Answer from the drawing. Dimensions are ordinates in mm from the lowest x, y and z of the part. A direction names the side the tool comes from. Coordinates: 2 decimals unless noted, no trailing zeros. Write each loop counter-clockwise with the first axis right and the second up, starting at its lowest first coordinate (ties: lowest second). Pieces come first, ordered by that corner, then holes. Notation, with made-up numbers: M 0.25,-16 L 47.25,-16 A19 ccw 47.25,-9 Z; hole C -9,-15 d8. An arc over 180 degrees is marked long. Put each result on its own line as item: value. Start each with the question number.
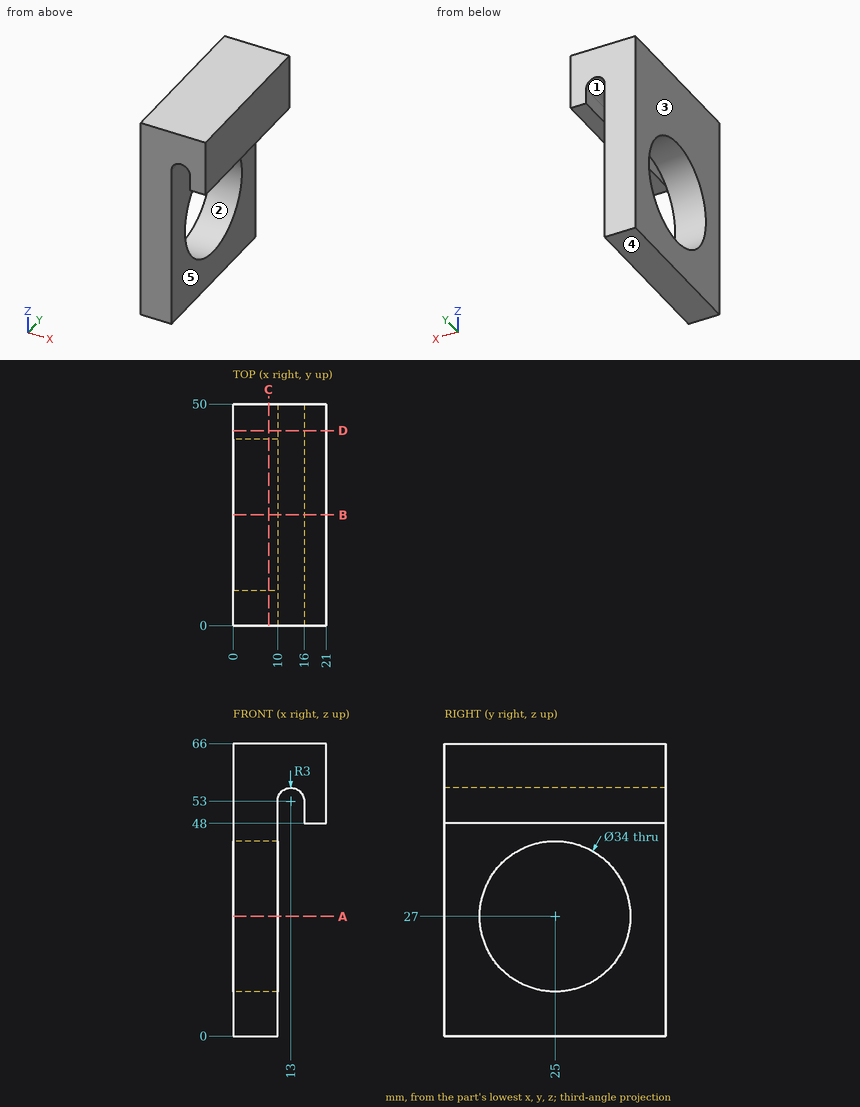
1) A cutting plane is placed at A-A on z = 27. Write down the section's boundary in (x, y), then the cut area to 3 significant figures.
2) For the marked faces 4 and 5, determine the directions among +Z, -Z, +X, -X, +Y, -Y from which every point of the face is accessible in a straight line to the end or side of a thin tool.
3) Given pin 1 Ø20.5 at (y, z) = (25, 27) entering from -X; pin 2 Ø12 at (y, z) = (22.5, 41.5) entering from +X; pin 3 Ø4 at (x, y) = (17.5, 34.5) entering from -Z, each flat-ended and moving along its own axis, determine where each tip first touches the part or whether it passes through.
4) A cutting plane is placed at B-B on y = 25. Write down the section's boundary in (x, z).
5) Determine the mould class of the marked faces 1, 2 and 3 for opening direction Z: +Z half, -Z half, draft (parallel to the pull), parting line (faces both ways), or undercut.
6) A cutting plane is placed at C-C on x = 8. Write down the section's boundary in (y, z).
7) Straight lines are drawn through the part: probe 1 along Z at (x, y) = (4.5, 25); probe 2 along X at (y, z) = (31, 53); probe 3 along Z at (x, y) = (2, 29). For each, find the intervals that lie inside material, in ascending order.
8) A cutting plane is placed at D-D on y = 44. Write down the section's boundary in (x, z), then the cut area to 3 significant figures.
Answers follow:
1. outline: M 0,0 L 10,0 L 10,8 L 0,8 Z; M 0,42 L 10,42 L 10,50 L 0,50 Z
1. area: 160 mm²
2. face 4: -Z, +X, -X, +Y, -Y
2. face 5: -Z, +Y, -Y
3. pin 1: passes through
3. pin 2: stops at x = 10
3. pin 3: stops at z = 48
4. outline: M 0,0 L 10,0 L 10,10 L 0,10 Z; M 0,44 L 10,44 L 10,53 A3 cw 16,53 L 16,48 L 21,48 L 21,66 L 0,66 Z
5. face 1: -Z half
5. face 2: undercut
5. face 3: draft
6. outline: M 0,0 L 50,0 L 50,66 L 0,66 Z; hole C 25,27 d34
7. probe 1: z = 0 to 10, 44 to 66
7. probe 2: x = 0 to 10, 16 to 21
7. probe 3: z = 0 to 10.48, 43.52 to 66
8. outline: M 0,0 L 10,0 L 10,53 A3 cw 16,53 L 16,48 L 21,48 L 21,66 L 0,66 Z
8. area: 814 mm²
